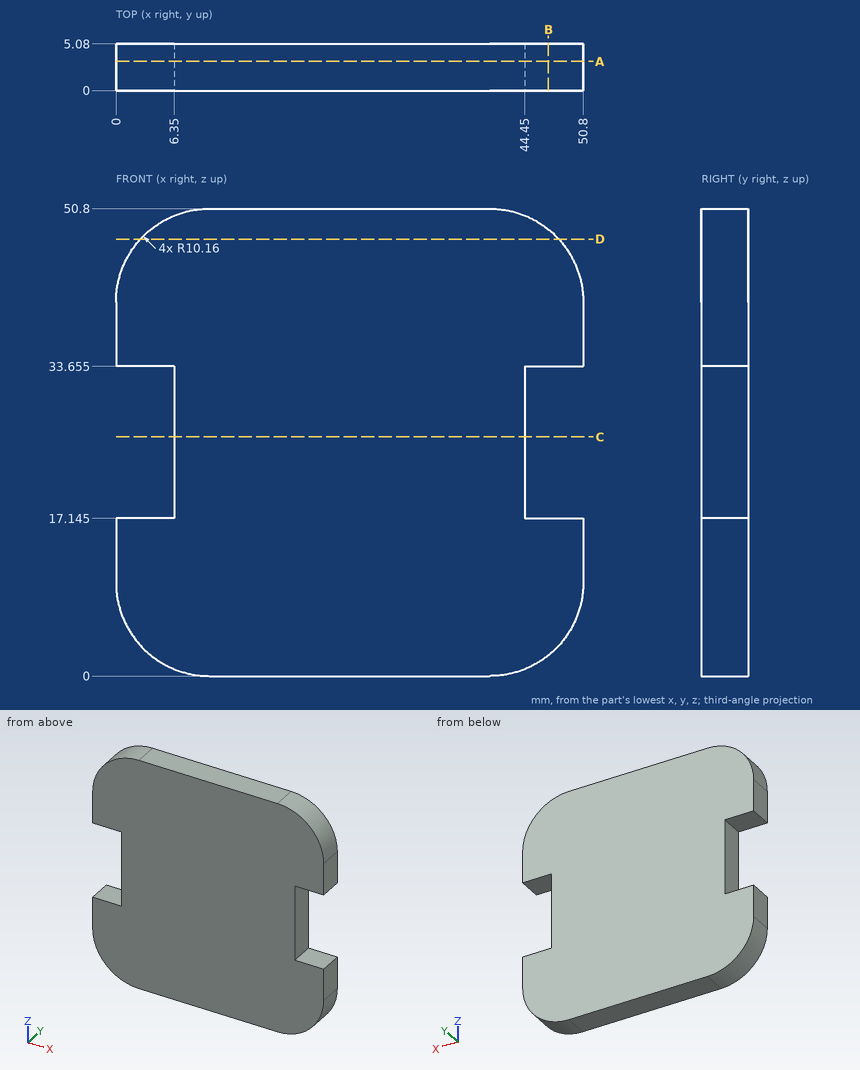
Source: three-view drawing plus pictorial views. Frame: mm from the lowest corner of the part. Round coordinates to 2 decimals unless told otherwise and drop trailing zeros. Loops run counter-clockwise (first coordinate to the right, second up) from the corner with the lowest first, then second, coordinate; pieces in that order, holes last.
Item 1: Section B-B, the plane x = 47. Output: boundary loops of the cut face in (y, z) (3 decimals).
Checked values:
outline: (0, 2.237) - (5.08, 2.237) - (5.08, 17.145) - (0, 17.145) - close; (0, 33.655) - (5.08, 33.655) - (5.08, 48.563) - (0, 48.563) - close
Item 2: Section A-A, the plane y = 3.2. Output: boundary loops of the cut face in (x, z) (3 decimals), plus the area to 3 significant figures.
Checked values:
outline: (0, 10.16) arc R10.16 ccw to (10.16, 0) - (40.64, 0) arc R10.16 ccw to (50.8, 10.16) - (50.8, 17.145) - (44.45, 17.145) - (44.45, 33.655) - (50.8, 33.655) - (50.8, 40.64) arc R10.16 ccw to (40.64, 50.8) - (10.16, 50.8) arc R10.16 ccw to (0, 40.64) - (0, 33.655) - (6.35, 33.655) - (6.35, 17.145) - (0, 17.145) - close
area: 2,280 mm2
Item 3: Line query: L1, parallel to X at y = 3.4, z = 22; L2, parallel to Z at x = 2, y = 4.8 (3 decimals); L3, parallel to Z at x = 7.5, y = 1.2. Output: solid intervals per line, ascending.
Checked values:
L1: x = 6.35 to 44.45
L2: z = 4.107 to 17.145, 33.655 to 46.693
L3: z = 0.35 to 50.45
Item 4: Section D-D, the plane z = 47.5. Output: boundary loops of the cut face in (x, y).
Checked values:
outline: (2.67, 0) - (48.13, 0) - (48.13, 5.08) - (2.67, 5.08) - close
Item 5: Section C-C, the plane z = 26. Output: boundary loops of the cut face in (x, y).
Checked values:
outline: (6.35, 0) - (44.45, 0) - (44.45, 5.08) - (6.35, 5.08) - close
Item 6: Contact query for flat-ended pins moving along their axis: P1, Ø2.5, axis at y = 3, z = 22, coming from the +X side; P2, Ø3, axis at y = 1, z = 30, coming from the -X side; P3, Ø2.5, axis at x = 49, y = 3, coming from the +Z side. Output: stop coordinate, or through.
Checked values:
P1: stops at x = 44.45
P2: stops at x = 6.35
P3: stops at z = 47.9
